Check sheet for the modelled part. Datum: model origin and axes. Units: mm. Face numbers are marked on the shaded views. A direction names the side the tool comes from. Coordinates: 2 decimals unless noted, no trailing zeros. Order: outer loops, then holes, each group sorted by start corner. A loop starts at its lowest first (then second) coordinate and runs counter-clockwise, first axis right, second up. Notation, with made-up numbers: M 64.25,50.5 L 86.25,50.5 A28 ccw 86.25,69.5 Z; hole C 40.25,-40 d8. An arc over 180 degrees is marked long. Answer in a Markdown table with one row per item. Add a question column.
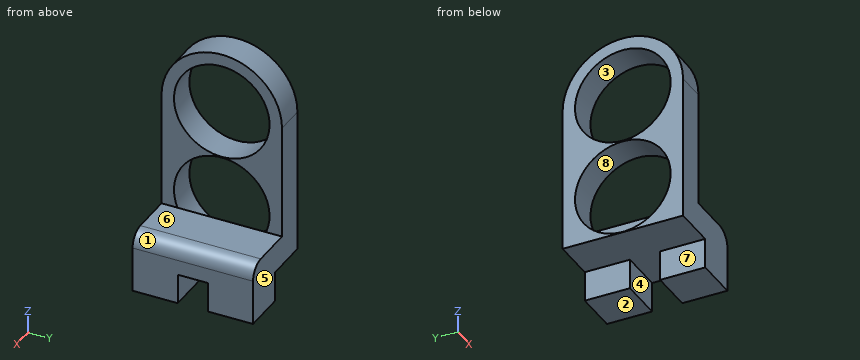
from build123d import *

# Parameters (mm, degrees)
F1_DEPTH  = 2
F2_W      = 8
F2_H      = 2
F3_DEPTH  = 3.75
F4_W      = 2.875
F4_H      = 8
F5_DEPTH  = 2
F6_W      = 2
F6_H      = 2
F7_DEPTH  = 25
F8_R      = 3.175
F9_DEPTH  = 2
F10_R     = 3.175
F11_DEPTH = 2
F12_R     = 1


with BuildPart() as f1:
    # F0 (on Right) → F1 (new body)
    with BuildSketch(Plane.YZ):
        with BuildLine():
            Line((-4, 9.6), (4, 9.6))
            ThreePointArc((4, 9.6), (0, 13.6), (-4, 9.6))
        make_face()
        with BuildLine():
            ThreePointArc((-4, 9.6), (0, 5.6), (4, 9.6))
            Line((4, 9.6), (-4, 9.6))
        make_face()
        with BuildLine():
            Line((4, 0), (4, 9.6))
            ThreePointArc((4, 9.6), (0, 5.6), (-4, 9.6))
            Line((-4, 9.6), (-4, 0))
            Line((-4, 0), (4, 0))
        make_face()
    extrude(amount=F1_DEPTH)

    # F2 (on face) → F3 (join)
    with BuildSketch(Plane.YZ.offset(2)):
        with Locations((0, 1)):
            Rectangle(F2_W, F2_H)
    extrude(amount=F3_DEPTH)

    # F4 (on face) → F5 (join)
    with BuildSketch(Plane(origin=(0, 0, 0), x_dir=(1, 0, 0), z_dir=(0, 0, -1))):
        with Locations((4.3125, 0)):
            Rectangle(F4_W, F4_H)
    extrude(amount=F5_DEPTH)

    # F6 (on face) → F7 (cut)
    with BuildSketch(Plane.YZ.offset(5.75)):
        with Locations((0, -1)):
            Rectangle(F6_W, F6_H)
    extrude(amount=-F7_DEPTH, mode=Mode.SUBTRACT)

    # F8 (on face) → F9 (cut)
    with BuildSketch(Plane(origin=(0, 0, 0), x_dir=(0, -1, 0), z_dir=(-1, 0, 0))):
        with Locations((0, 9.6)):
            Circle(F8_R)
    extrude(amount=-F9_DEPTH, mode=Mode.SUBTRACT)

    # F10 (on face) → F11 (cut)
    with BuildSketch(Plane(origin=(0, 0, 0), x_dir=(0, -1, 0), z_dir=(-1, 0, 0))):
        with Locations((0, 3.2)):
            Circle(F10_R)
    extrude(amount=-F11_DEPTH, mode=Mode.SUBTRACT)

    # F12
    f12_edges = [f1.edges().sort_by_distance(p)[0] for p in [
        (5.75, 0, 2),
    ]]
    fillet(f12_edges, radius=F12_R)


solid = f1.part
1. Set-up check for the marked faces 4, 5, 6, 7 and 8: record each of +Z, -Z, +X, -X, +Y, -Y from which the full face is reachable in a straight line by a thin tool's end or side.
2. Release check for a two-part mould opening along Z. For the marked faces 1, 2 and 3 record: released by +Z, released by -Z, zero draft, split by the parting line, or undercut.
3. Section check A-A on z = 3.2. Enter the section's corners in (x, y) (3 decimals), then the cut area to 3 significant figures.
4. Scan lines: line 1 (Z direction, x = 0.55, y = -2.5); line 2 (Y direction, x = 5.1, z = -1); line 3 (Z direction, x = 3.75, y = 1.5). Record each from-to range of solid material in increasing order.
5. Go/stop test with flat-tipped pins: pin 1 Ø3 at (x, y) = (3, -1.5) entering from +Z; pin 2 Ø4 at (y, z) = (0.5, 5) entering from +X; pin 3 Ø0.6 at (y, z) = (-1, 1.5) entering from -X; pin 4 Ø4 at (y, z) = (0, 9.6) entering from -X. Record where each tip stops, or that it passes through.
6. Section check D-D on x = 1.2. Enter the section's corners in (y, z) (3 decimals).
7. Section check B-B on y = 0. Enter the section's corners in (x, z) (3 decimals), then the cut area to 3 significant figures.
8. Section check C-C on x = 4.45. Enter the section's corners in (y, z), then the cut area to 3 significant figures.
Result sheet:
| question | item | result |
|---|---|---|
| 1 | face 4 | -Z, +X, -X |
| 1 | face 5 | +Z, -Z, +X, -X, +Y |
| 1 | face 6 | +Z, +X, +Y, -Y |
| 1 | face 7 | -Z, -X, +Y, -Y |
| 1 | face 8 | -X |
| 2 | face 1 | released by +Z |
| 2 | face 2 | released by -Z |
| 2 | face 3 | undercut |
| 3 | outline | M 0,-4 L 2,-4 L 2,-3.175 L 0,-3.175 Z; M 0,3.175 L 2,3.175 L 2,4 L 0,4 Z |
| 3 | area | 3.30 mm^2 |
| 4 | line 1 | 0 to 1.24, 5.16 to 7.64, 11.56 to 12.72 |
| 4 | line 2 | -4 to -1, 1 to 4 |
| 4 | line 3 | -2 to 2 |
| 5 | pin 1 | z = 13.58 |
| 5 | pin 2 | x = 2 |
| 5 | pin 3 | x = 2 |
| 5 | pin 4 | through |
| 6 | outline | M -4,0 L 4,0 L 4,9.6 A4 ccw -4,9.6 Z; hole C 0,3.2 d6.35; hole C 0,9.6 d6.35 |
| 7 | outline | M 0,0 L 5.75,0 L 5.75,1 A1 ccw 4.75,2 L 2,2 L 2,0.025 L 0,0.025 Z; M 0,6.375 L 2,6.375 L 2,6.425 L 0,6.425 Z; M 0,12.775 L 2,12.775 L 2,13.6 L 0,13.6 Z |
| 7 | area | 9.09 mm^2 |
| 8 | outline | M -4,-2 L -1,-2 L -1,0 L 1,0 L 1,-2 L 4,-2 L 4,2 L -4,2 Z |
| 8 | area | 28.0 mm^2 |
